```python
from build123d import *

# Parameters (mm, degrees)
BOX003_W                 = 14
BOX003_H                 = 1
BOX003_DEPTH             = 1
ARRAY001_Y_COUNT         = 5
ARRAY001_Y_PITCH         = 2
ARRAY001_PLACEMENT_ANGLE = 90
BOX002_W                 = 14
BOX002_H                 = 1
BOX002_DEPTH             = 1
ARRAY_Y_COUNT            = 5
ARRAY_Y_PITCH            = 2
BOX001_W                 = 10
BOX001_H                 = 10
BOX001_DEPTH             = 8
BOX_W                    = 12
BOX_H                    = 12
BOX_DEPTH                = 18


with BuildPart() as array001:
    # Box003 → Box003 (new body)
    with BuildSketch(Plane.XY):
        with Locations((7, 0.5)):
            Rectangle(BOX003_W, BOX003_H)
    extrude(amount=BOX003_DEPTH)

    # Array001 Y: Array001 ×5


with BuildPart() as array001_1:
    add(array001.part)
    with Locations(*[(0, i * ARRAY001_Y_PITCH, 0) for i in range(1, ARRAY001_Y_COUNT)]):
        add(array001.part)


with BuildPart() as array001_2:
    # Array001 placement: moved
    add(array001_1.part.moved(Location((10.5, -1.5, 17))).rotate(Axis((10.5, -1.5, 17), (0, 0, 1)), ARRAY001_PLACEMENT_ANGLE))


with BuildPart() as array:
    # Box002 → Box002 (new body)
    with BuildSketch(Plane.XY):
        with Locations((7, 0.5)):
            Rectangle(BOX002_W, BOX002_H)
    extrude(amount=BOX002_DEPTH)

    # Array Y: Array ×5


with BuildPart() as array_1:
    add(array.part)
    with Locations(*[(0, i * ARRAY_Y_PITCH, 0) for i in range(1, ARRAY_Y_COUNT)]):
        add(array.part)


with BuildPart() as array_2:
    # Array placement: moved
    add(array_1.part.moved(Location((-1, 2, 17))))


with BuildPart() as cub001:
    # Box001 → Box001 (new body)
    with BuildSketch(Plane(origin=(1, 1, 15), x_dir=(1, 0, 0), z_dir=(0, 0, 1))):
        with Locations((5, 5)):
            Rectangle(BOX001_W, BOX001_H)
    extrude(amount=BOX001_DEPTH)


with BuildPart() as cut002:
    # Box → Box (new body)
    with BuildSketch(Plane.XY):
        with Locations((6, 6)):
            Rectangle(BOX_W, BOX_H)
    extrude(amount=BOX_DEPTH)

    # Cut: cut Cub001
    add(cub001.part, mode=Mode.SUBTRACT)

    # Cut001: cut Array
    add(array_2.part, mode=Mode.SUBTRACT)

    # Cut002: cut Array001
    add(array001_2.part, mode=Mode.SUBTRACT)


solid = cut002.part
```
Part model, mm, in its own coordinate system. A direction names the side the tool comes from. Round coordinates to 2 decimals unless told otherwise and drop trailing zeros. Loops run counter-clockwise (first coordinate to the right, second up) from the corner with the lowest first, then second, coordinate; pieces in that order, holes last.
1. Slice it at B-B (z = 16.5). Give the cut face in (x, y), and give its area (3 significant figures).
Solutions:
outline: (0, 0) - (12, 0) - (12, 12) - (0, 12) - close; hole (1, 1) - (11, 1) - (11, 11) - (1, 11) - close
area: 44.0 mm2
2. Slice it at A-A (x = 9.75). Give the cut face in (y, z).
Solutions:
outline: (0, 0) - (12, 0) - (12, 17) - (11, 17) - (11, 15) - (1, 15) - (1, 17) - (0, 17) - close
3. 3-axis set-ups, long thin cutter, end or side, ignore diameter. For faces 1 (the face through (11.5, 5, 17.5)), 2 (the face through (0.7, 11.5, 18)), 3 (the face through (7.5, 11.5, 17.5)): which of +Z, -Z, +X, -X, +Y, -Y reach the whole face in a straight line?
Solutions:
face 1: +Z, +X, -X
face 2: +Z, +X, -X, +Y, -Y
face 3: +Z, +Y, -Y
4. Slice it at C-C (y = 5.5). Give the cut face in (x, z), and give its area (3 significant figures).
Solutions:
outline: (0, 0) - (12, 0) - (12, 18) - (11, 18) - (11, 15) - (1, 15) - (1, 18) - (0, 18) - close
area: 186 mm2
5. Flat gauge pins, fed straight in: pin 1 (0.5 mm diameter, centred on x = 0.5, y = 8.5, fed in from +Z); pin 2 (2 mm diameter, centred on x = 4, y = 6, fed in from +Z). Where does each tip first touch, or does it go through?
Solutions:
pin 1: stops at z = 17
pin 2: stops at z = 15
6. Two-plate mould, pull along X, no slides. Class faces 4 (the face through (5, 0.5, 18)), 5 (the face through (3.5, 0.5, 17.5)): pulls with the +X half, pulls with the -X half, needs draft (parallel to the pull), parting line crosses it, or undercut.
Solutions:
face 4: needs draft
face 5: undercut
7. Drill centre lines: line 1 along X through (y, z) = (6.5, 15.75); line 2 along Z through (x, y) = (10, 4); line 3 along Z through (x, y) = (7.75, 11.25). Where is each one in solid material? Low to high.
Solutions:
line 1: x = 0 to 1, 11 to 12
line 2: z = 0 to 15
line 3: z = 0 to 17
